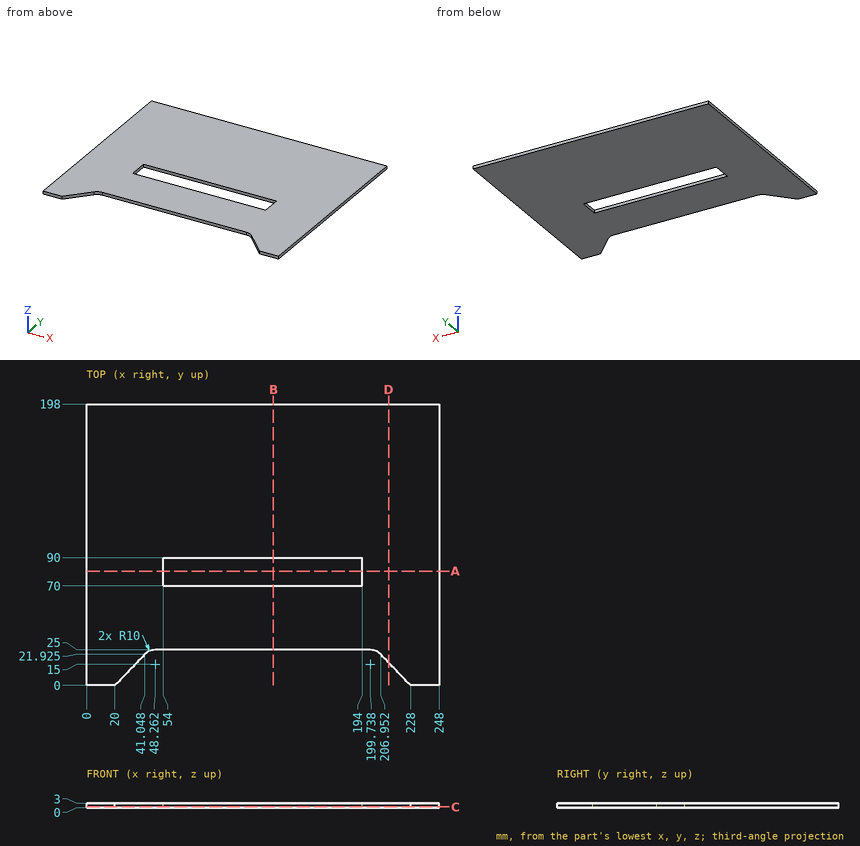
The drawing under review shows one solid part. Ordinate dimensions are in mm from its lowest x, y, z. Round coordinates to 2 decimals unless told otherwise and drop trailing zeros. Write each loop counter-clockwise with the first axis right and the second up, starting at its lowest first coordinate (ties: lowest second). Pieces come first, ordered by that corner, then holes. Notation, with made-up numbers: (0.5, 65) -> (11.5, 65) arc R20 ccw to (11.5, 104) -> close; hole circle Ø1 at (73.25, 43.5). An arc over 180 degrees is marked (long way). One line per question, with ' | ' between items. Start each with the question number.
(1) Add section C-C, the plane z = 0.6. Write out the cut boundary in (x, y) (1 decimal).
(2) For line 1 along Y through (x, z) = (80, 0.45); line 2 along X through (y, z) = (73.5, 2.6); line 3 along X through (y, z) = (15, 2.65), list the stretches that pass through material, from the lowest coordinate up. Write a range as from..to.
(3) Add section A-A, the plane y = 80.5. Write out the cut boundary in (x, z), plus the area to 3 significant figures.
(4) Add section D-D, the plane x = 212.5. Write out the cut boundary in (y, z).
(5) Add section B-B, the plane x = 131.5. Write out the cut boundary in (y, z), plus the area to 3 significant figures.
Answer list:
1) outline: (0, 0) -> (20, 0) -> (41, 21.9) arc R10 cw to (48.3, 25) -> (199.7, 25) arc R10 cw to (207, 21.9) -> (228, 0) -> (248, 0) -> (248, 198) -> (0, 198) -> close; hole (54, 70) -> (194, 70) -> (194, 90) -> (54, 90) -> close
2) line 1: 25..70, 90..198 | line 2: 0..54, 194..248 | line 3: 0..34.4, 213.6..248
3) outline: (0, 0) -> (54, 0) -> (54, 3) -> (0, 3) -> close; (194, 0) -> (248, 0) -> (248, 3) -> (194, 3) -> close | area: 324 mm²
4) outline: (16.15, 0) -> (198, 0) -> (198, 3) -> (16.15, 3) -> close
5) outline: (25, 0) -> (70, 0) -> (70, 3) -> (25, 3) -> close; (90, 0) -> (198, 0) -> (198, 3) -> (90, 3) -> close | area: 459 mm²
